from build123d import *

# Parameters (mm, degrees)
SKETCH1_W           = 130
SKETCH1_H           = 40
BOSS_EXTRUDE1_DEPTH = 6
SKETCH2_W           = 12.3
SKETCH2_H           = 12.3
BOSS_EXTRUDE2_DEPTH = 10
LPATTERN1_COUNT     = 4
LPATTERN1_PITCH     = 30
CHAMFER1_SIZE       = 0.5


with BuildPart() as part:
    # Sketch1 → Boss-Extrude1 (new body)
    with BuildSketch(Plane(origin=(0, 0, 0), x_dir=(1, 0, 0), z_dir=(0, 1, 0))):
        Rectangle(SKETCH1_W, SKETCH1_H)
    extrude(amount=BOSS_EXTRUDE1_DEPTH)

    # Sketch2 → Boss-Extrude2 (add)
    with BuildSketch(Plane.XZ):
        with Locations((-45, 0)):
            Rectangle(SKETCH2_W, SKETCH2_H)
    boss_extrude2 = extrude(amount=BOSS_EXTRUDE2_DEPTH)

    # LPattern1: Boss-Extrude2 ×4
    with Locations(*[(i * LPATTERN1_PITCH, 0, 0) for i in range(1, LPATTERN1_COUNT)]):
        add(boss_extrude2)

    # Chamfer1
    chamfer1_edges = [part.edges().sort_by_distance(p)[0] for p in [
        (-51.15, -10, 0),
        (-45, -10, -6.15),
        (-38.85, -10, 0),
        (-45, -10, 6.15),
        (-21.15, -10, 0),
        (-15, -10, -6.15),
        (-8.85, -10, 0),
        (-15, -10, 6.15),
        (8.85, -10, 0),
        (15, -10, -6.15),
        (21.15, -10, 0),
        (15, -10, 6.15),
        (38.85, -10, 0),
        (45, -10, -6.15),
        (51.15, -10, 0),
        (45, -10, 6.15),
    ]]
    chamfer(chamfer1_edges, length=CHAMFER1_SIZE)


solid = part.part
Build history of the part. All positions in model axes, mm. A direction names the side the tool comes from. Round coordinates to 2 decimals unless told otherwise and drop trailing zeros. Write each loop counter-clockwise with the first axis right and the second up, starting at its lowest first coordinate (ties: lowest second). Pieces come first, ordered by that corner, then holes. Notation, with made-up numbers: (18.5, -11) -> (62.5, -11) arc R27 cw to (62.5, 21) -> close; hole circle Ø2 at (38.5, 37). An arc over 180 degrees is marked (long way). Use one line per item in the form item = value.
Q1. Two-plate mould, pull along X, no slides. Class faces 1 (the flat face through (-65, 3, 0)), 2 (the flat face through (38.85, -5, 0)), 3 (the flat face through (65, 3, 0)), 4 (the flat face through (-1, 6, 0)): released by +X, released by -X, zero draft, split by the parting line, or undercut.
Conclusion:
face_1 = released by -X
face_2 = undercut
face_3 = released by +X
face_4 = zero draft
Q2. Tool access for faces 5 (the flat face through (15, -5, 6.15)), 6 (the flat face through (-45, -5, -6.15)), 7 (the flat face through (-38.85, -5, 0)): list every direction of +Z, -Z, +X, -X, +Y, -Y with a clear straight run to the whole face (end or side of a thin tool).
Conclusion:
face_5 = +Z, +X, -X, -Y
face_6 = -Z, +X, -X, -Y
face_7 = +Z, -Z, -Y
Q3. Band-saw the part on A-A, the plane y = -7.75. Write the cut outline in (x, z), then the cut area to 3 significant figures.
Conclusion:
outline = (-51.15, -6.15) -> (-38.85, -6.15) -> (-38.85, 6.15) -> (-51.15, 6.15) -> close; (-21.15, -6.15) -> (-8.85, -6.15) -> (-8.85, 6.15) -> (-21.15, 6.15) -> close; (8.85, -6.15) -> (21.15, -6.15) -> (21.15, 6.15) -> (8.85, 6.15) -> close; (38.85, -6.15) -> (51.15, -6.15) -> (51.15, 6.15) -> (38.85, 6.15) -> close
area = 605 mm²
Q4. Drill centre lines: L1, parallel to X at y = -3.25, z = 0; L2, parallel to Z at x = -19, y = -1. Where is each one in solid material? Low to high.
Conclusion:
L1 = -51.15 to -38.85, -21.15 to -8.85, 8.85 to 21.15, 38.85 to 51.15
L2 = -6.15 to 6.15
Q5. Band-saw the part on D-D, the plane z = 11.5. Write the cut outline in (x, y).
Conclusion:
outline = (-65, 0) -> (65, 0) -> (65, 6) -> (-65, 6) -> close
Q6. Band-saw the part on C-C, the plane z = -1. Write the cut outline in (x, y), then the cut area to 3 significant figures.
Conclusion:
outline = (-65, 0) -> (-51.15, 0) -> (-51.15, -9.5) -> (-50.65, -10) -> (-39.35, -10) -> (-38.85, -9.5) -> (-38.85, 0) -> (-21.15, 0) -> (-21.15, -9.5) -> (-20.65, -10) -> (-9.35, -10) -> (-8.85, -9.5) -> (-8.85, 0) -> (8.85, 0) -> (8.85, -9.5) -> (9.35, -10) -> (20.65, -10) -> (21.15, -9.5) -> (21.15, 0) -> (38.85, 0) -> (38.85, -9.5) -> (39.35, -10) -> (50.65, -10) -> (51.15, -9.5) -> (51.15, 0) -> (65, 0) -> (65, 6) -> (-65, 6) -> close
area = 1,270 mm²
Q7. Band-saw the part on B-B, the plane x = -13. Write the cut outline in (y, z), then the cut area to 3 significant figures.
Conclusion:
outline = (-10, -5.65) -> (-9.5, -6.15) -> (0, -6.15) -> (0, -20) -> (6, -20) -> (6, 20) -> (0, 20) -> (0, 6.15) -> (-9.5, 6.15) -> (-10, 5.65) -> close
area = 363 mm²
Q8. Drop flat-ended pins along their axis: P1, Ø7.5, axis at x = -14.5, y = -4.5, coming from the +Z side; P2, Ø5, axis at y = -5, z = 0, coming from the +X side; P3, Ø3, axis at y = -4, z = -1, coming from the -X side. Give the stop position or say it passes through.
Conclusion:
P1 = 6.15
P2 = 51.15
P3 = -51.15
